Input: dimensioned drawing with shaded views. Units: mm. Origin: part minimum x, y, z. A direction names the side the tool comes from. Coordinates: 2 decimals unless noted, no trailing zeros. Order: outer loops, then holes, each group sorted by start corner. A loop starts at its lowest first (then second) coordinate and runs counter-clockwise, first axis right, second up.
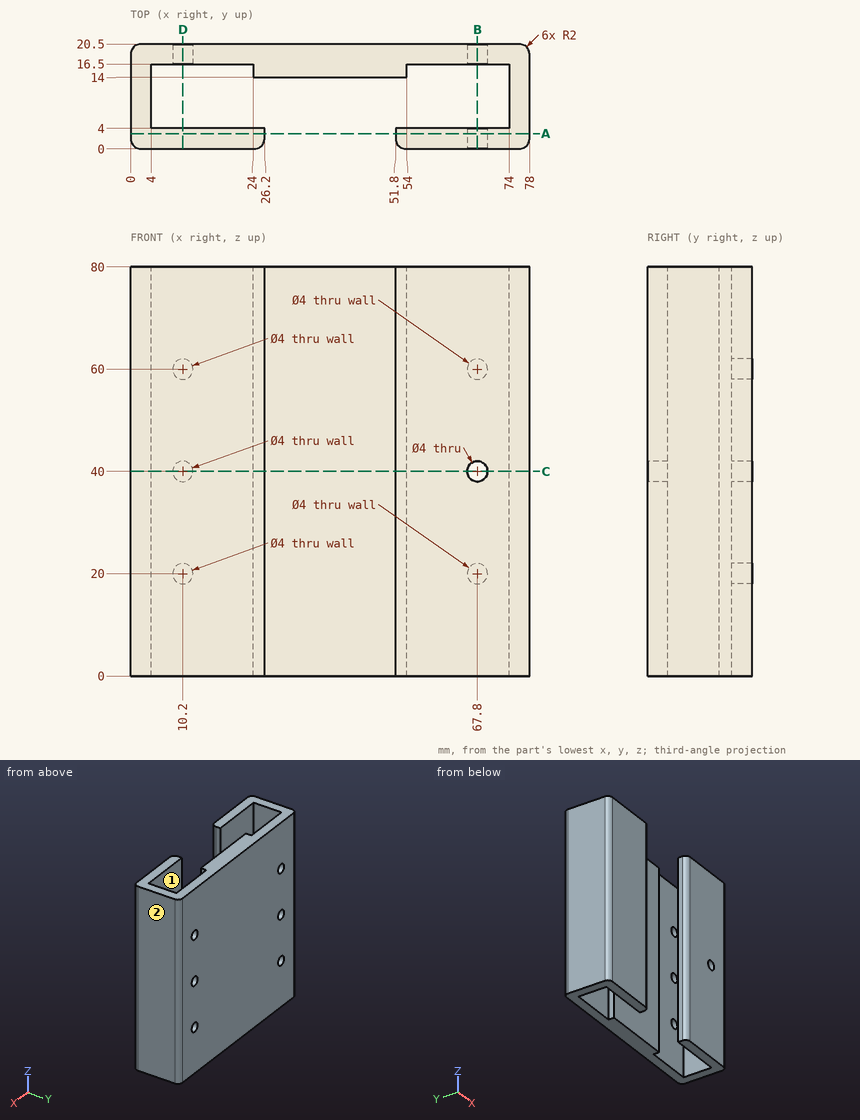
1. Section query D-D, the plane x = 10.2. Output: boundary loops of the cut face in (y, z), plus the area to 3 significant figures.
2. Contact query for a flat-ended pin moving along its axis: P1, Ø3.5, axis at x = 10.2, z = 60, coming from the +Y side. Output: stop coordinate, or through.
3. Section query C-C, the plane z = 40. Count the separate pieces of the cut face and the enclosed holes in it, plus the area to 3 significant figures.
4. Section query B-B, the plane x = 67.8. Output: boundary loops of the cut face in (y, z).
5. Material intervals for line 1 along Z through (x, y) = (67.8, 17.4); line 2 along X through (y, z) = (16, 71); line 3 along Y through (x, z) = (9.5, 50.5), sorted ascending.
6. Section query A-A, the plane y = 3. Output: boundary loops of the cut face in (x, z), plus the area to 3 significant figures.
7. Access query for the marked faces 1 and 2. Directions: +Z, -Z, +X, -X, +Y, -Y. A direction counts if a zero-diameter tool reaches every point of the face in a straight line with its end or side. Return the directions, or none.
Answer key:
1. outline: (0, 0) - (4, 0) - (4, 80) - (0, 80) - close; (16.5, 0) - (20.5, 0) - (20.5, 18) - (16.5, 18) - close; (16.5, 22) - (20.5, 22) - (20.5, 38) - (16.5, 38) - close; (16.5, 42) - (20.5, 42) - (20.5, 58) - (16.5, 58) - close; (16.5, 62) - (20.5, 62) - (20.5, 80) - (16.5, 80) - close
1. area: 592 mm2
2. P1: stops at y = 4
3. separate pieces: 4
3. enclosed holes: 0
3. area: 643 mm2
4. outline: (0, 0) - (4, 0) - (4, 38) - (0, 38) - close; (0, 42) - (4, 42) - (4, 80) - (0, 80) - close; (16.5, 0) - (20.5, 0) - (20.5, 18) - (16.5, 18) - close; (16.5, 22) - (20.5, 22) - (20.5, 38) - (16.5, 38) - close; (16.5, 42) - (20.5, 42) - (20.5, 58) - (16.5, 58) - close; (16.5, 62) - (20.5, 62) - (20.5, 80) - (16.5, 80) - close
5. line 1: z = 0 to 18, 22 to 38, 42 to 58, 62 to 80
5. line 2: x = 0 to 4, 24 to 54, 74 to 78
5. line 3: y = 0 to 4, 16.5 to 20.5
6. outline: (0, 0) - (26.2, 0) - (26.2, 80) - (0, 80) - close; (51.8, 0) - (78, 0) - (78, 80) - (51.8, 80) - close; hole circle Ø4 at (67.8, 40)
6. area: 4,180 mm2
7. face 1: +Z, -Z
7. face 2: +Z, -Z, +X, +Y, -Y
